```python
from build123d import *

# Parameters (mm, degrees)
F1_DEPTH = 3.175


with BuildPart() as f1:
    # F0 (on Top) → F1 (new body)
    with BuildSketch(Plane.XY):
        Polygon((-63.146477, 115.279474), (-63.146477, 127.979474), (-63.146477, 204.179474), (-66.321477, 204.179474), (-66.321477, 115.279474), align=None)
        Polygon((-56.161477, 204.179474), (-56.161477, 127.979474), (-56.161477, 115.279474), (-52.986477, 115.279474), (-52.986477, 204.179474), align=None)
        Polygon((-56.161477, 127.979474), (-63.146477, 127.979474), (-63.146477, 115.279474), (-63.146477, -37.120526), (-56.161477, -37.120526), (-56.161477, 115.279474), align=None)
    extrude(amount=F1_DEPTH)


solid = f1.part
```
Input: part model. Units: mm. Frame: model coordinates. Coordinates: 2 decimals unless noted, no trailing zeros. Write each loop counter-clockwise with the first axis right and the second up, starting at its lowest first coordinate (ties: lowest second). Pieces come first, ordered by that corner, then holes.
1) Section D-D on y = 99. Output: boundary loops of the cut face in (x, z) (3 decimals), and give its area (3 significant figures).
2) Section C-C on x = -60.25. Output: boundary loops of the cut face in (y, z) (3 decimals), and give its area (3 significant figures).
3) Section B-B on z = 2. Output: boundary loops of the cut face in (x, y), and give its area (3 significant figures).
4) Section A-A on y = 161.5. Output: boundary loops of the cut face in (x, z) (3 decimals), and give its area (3 significant figures).
5) Pin query (flat end, axial travel): pin 1 Ø1 at (x, z) = (-54, 1.5) entering from -Y; pin 2 Ø1.5 at (x, z) = (-57.5, 2) entering from +Y; pin 3 Ø1.6 at (y, z) = (29.5, 1.5) entering from -X. Return the tip coordinate at first contact, or that it passes through.
6) Material intervals for line 1 along X through (y, z) = (168, 0.45); line 2 along Y through (x, z) = (-63.25, 2.1); line 3 along X through (y, z) = (93.5, 2.05), sorted ascending.
Check result:
1. outline: (-63.146, 0) - (-56.161, 0) - (-56.161, 3.175) - (-63.146, 3.175) - close
1. area: 22.2 mm2
2. outline: (-37.121, 0) - (127.979, 0) - (127.979, 3.175) - (-37.121, 3.175) - close
2. area: 524 mm2
3. outline: (-66.32, 115.28) - (-63.15, 115.28) - (-63.15, -37.12) - (-56.16, -37.12) - (-56.16, 115.28) - (-52.99, 115.28) - (-52.99, 204.18) - (-56.16, 204.18) - (-56.16, 127.98) - (-63.15, 127.98) - (-63.15, 204.18) - (-66.32, 204.18) - close
3. area: 1,720 mm2
4. outline: (-66.321, 0) - (-63.146, 0) - (-63.146, 3.175) - (-66.321, 3.175) - close; (-56.161, 0) - (-52.986, 0) - (-52.986, 3.175) - (-56.161, 3.175) - close
4. area: 20.2 mm2
5. pin 1: stops at y = 115.28
5. pin 2: stops at y = 127.98
5. pin 3: stops at x = -63.15
6. line 1: x = -66.32 to -63.15, -56.16 to -52.99
6. line 2: y = 115.28 to 204.18
6. line 3: x = -63.15 to -56.16
